Source: CAD feature listing. Evaluate the final solid. Frame: model axes, mm. Face numbers are marked on the shaded views. Give positions to 0.01 mm unless a question says otherwise; leave off trailing zeros. Loops run counter-clockwise (first coordinate to the right, second up) from the corner with the lowest first, then second, coordinate; pieces in that order, holes last. Notation, with made-up numbers: M 0,2.25 L 18,2.25 A24 ccw 18,18.25 Z; hole C -32.75,-31.5 d1. An arc over 180 degrees is marked long. Answer in a Markdown table with one row per item.
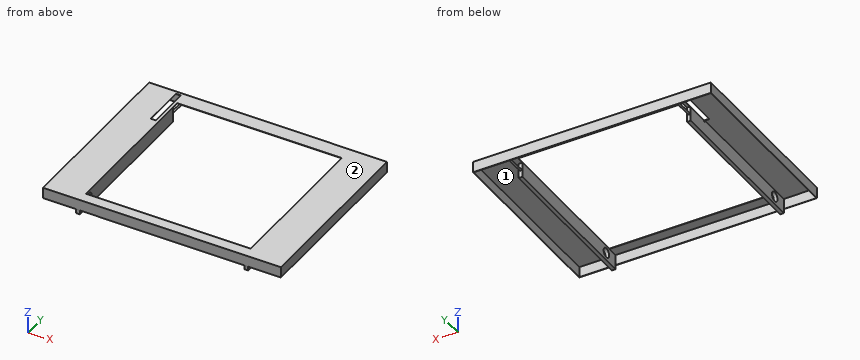
```python
from build123d import *

# Parameters (mm, degrees)
SKETCH1_W           = 650
SKETCH1_H           = 500
SKETCH1_W_2         = 450
SKETCH1_H_2         = 420
BOSS_EXTRUDE1_DEPTH = 15
SHELL1_T            = -1
SKETCH3_W           = 450
SKETCH3_H           = 10
CUT_EXTRUDE1_DEPTH  = 20
SKETCH4_W           = 10
SKETCH4_H           = 439
BOSS_EXTRUDE2_DEPTH = 41
SKETCH5_R           = 13
CUT_EXTRUDE2_DEPTH  = 470
SKETCH6_R           = 2.5
BOSS_EXTRUDE3_DEPTH = 50
SKETCH7_W           = 14
SKETCH7_H           = 119
CUT_EXTRUDE3_DEPTH  = 5


with BuildPart() as part:
    # Sketch1 → Boss-Extrude1 (new, symmetric)
    with BuildSketch(Plane.XY):
        Rectangle(SKETCH1_W, SKETCH1_H)
        Rectangle(SKETCH1_W_2, SKETCH1_H_2, mode=Mode.SUBTRACT)
    extrude(amount=BOSS_EXTRUDE1_DEPTH, both=True)

    # Shell1
    shell1_openings = [part.faces().sort_by_distance(p)[0] for p in [
        (0, -241.799390267, -15),
        (-225, 0, 0),
        (0, -210, 0),
        (225, 0, 0),
        (0, 210, 0),
    ]]
    offset(amount=SHELL1_T, openings=shell1_openings, kind=Kind.INTERSECTION)

    # Sketch3 → Cut-Extrude1 (cut, symmetric)
    with BuildSketch(Plane.XY):
        with Locations((0, -215)):
            Rectangle(SKETCH3_W, SKETCH3_H)
    extrude(amount=CUT_EXTRUDE1_DEPTH, both=True, mode=Mode.SUBTRACT)

    # Sketch4 → Boss-Extrude2 (add)
    with BuildSketch(Plane(origin=(0, 0, 14), x_dir=(-1, 0, 0), z_dir=(0, 0, -1))):
        with Locations((230, -29.5)):
            Rectangle(SKETCH4_W, SKETCH4_H)
    boss_extrude2 = extrude(amount=BOSS_EXTRUDE2_DEPTH)

    # Mirror1: Boss-Extrude2 across plane
    add(boss_extrude2.mirror(Plane(origin=(0, 0, 0), x_dir=(0, 0, 1), z_dir=(1, 0, 0))))

    # Sketch5 → Cut-Extrude2 (cut)
    with BuildSketch(Plane.ZY.offset(235)):
        with Locations((-5.5, -206)):
            Circle(SKETCH5_R)
    extrude(amount=-CUT_EXTRUDE2_DEPTH, mode=Mode.SUBTRACT)

    # Sketch6 → Boss-Extrude3 (add)
    with BuildSketch(Plane(origin=(0, 190, 0), x_dir=(1, 0, 0), z_dir=(0, 1, 0))):
        with Locations(Location((230, 5.5, 0), (0, 0, 180))):
            Circle(SKETCH6_R)
    boss_extrude3 = extrude(amount=BOSS_EXTRUDE3_DEPTH)

    # Mirror2: Boss-Extrude3 across plane
    add(boss_extrude3.mirror(Plane(origin=(0, 0, 0), x_dir=(0, 0, 1), z_dir=(1, 0, 0))))

    # Sketch7 → Cut-Extrude3 (cut)
    with BuildSketch(Plane.XY.offset(15)):
        with Locations((-240, 182.5)):
            Rectangle(SKETCH7_W, SKETCH7_H)
    extrude(amount=-CUT_EXTRUDE3_DEPTH, mode=Mode.SUBTRACT)


solid = part.part
```
1) Section D-D, the plane y = 34. Return loops of the section in (x, z), then the cut area to 3 significant figures.
Reply:
| item | result |
|---|---|
| outline | M -325,-15 L -324,-15 L -324,14 L -235,14 L -235,-27 L -225,-27 L -225,15 L -325,15 Z; M 225,-27 L 235,-27 L 235,14 L 324,14 L 324,-15 L 325,-15 L 325,15 L 225,15 Z |
| area | 1,080 mm² |
2) Section C-C, the plane x = 262.5. Return loops of the section in (y, z), then the cut area to 3 significant figures.
Reply:
| item | result |
|---|---|
| outline | M -250,-15 L -249,-15 L -249,14 L 249,14 L 249,-15 L 250,-15 L 250,15 L -250,15 Z |
| area | 558 mm² |
3) Pin query (flat end, axial travel): pin 1 Ø2 at (y, z) = (169, -17) entering from +X; pin 2 Ø8 at (x, z) = (227.5, -23) entering from -Y. Return the tip coordinate at first contact, or that it passes through.
Reply:
| item | result |
|---|---|
| pin 1 | stops at x = 235 |
| pin 2 | stops at y = -249 |
4) Pull-direction query (Y, two-part tool) for the marked faces 1 and 2; classes: released by +Y, released by -Y, zero draft, split by the parting line, or undercut.
Reply:
| item | result |
|---|---|
| face 1 | undercut |
| face 2 | zero draft |
5) Material intervals for L1, parallel to X at y = -80, z = 5.5; L2, parallel to Y at x = 230.5, z = -5.5; L3, parallel to X at y = 161, z = -23.5, sorted ascending.
Reply:
| item | result |
|---|---|
| L1 | x = -325 to -324, -235 to -225, 225 to 235, 324 to 325 |
| L2 | y = -250 to -219, -193 to 240, 249 to 250 |
| L3 | x = -235 to -225, 225 to 235 |
6) Section A-A, the plane x = 97.5. Return loops of the section in (y, z), then the cut area to 3 significant figures.
Reply:
| item | result |
|---|---|
| outline | M -250,-15 L -249,-15 L -249,14 L -220,14 L -220,15 L -250,15 Z; M 210,14 L 249,14 L 249,-15 L 250,-15 L 250,15 L 210,15 Z |
| area | 128 mm² |
7) Section B-B, the plane y = -206. Return loops of the section in (x, z).
Reply:
| item | result |
|---|---|
| outline | M -325,-15 L -324,-15 L -324,14 L -235,14 L -235,7.5 L -225,7.5 L -225,15 L -325,15 Z; M -235,-27 L -225,-27 L -225,-18.5 L -235,-18.5 Z; M 225,-27 L 235,-27 L 235,-18.5 L 225,-18.5 Z; M 225,7.5 L 235,7.5 L 235,14 L 324,14 L 324,-15 L 325,-15 L 325,15 L 225,15 Z |
